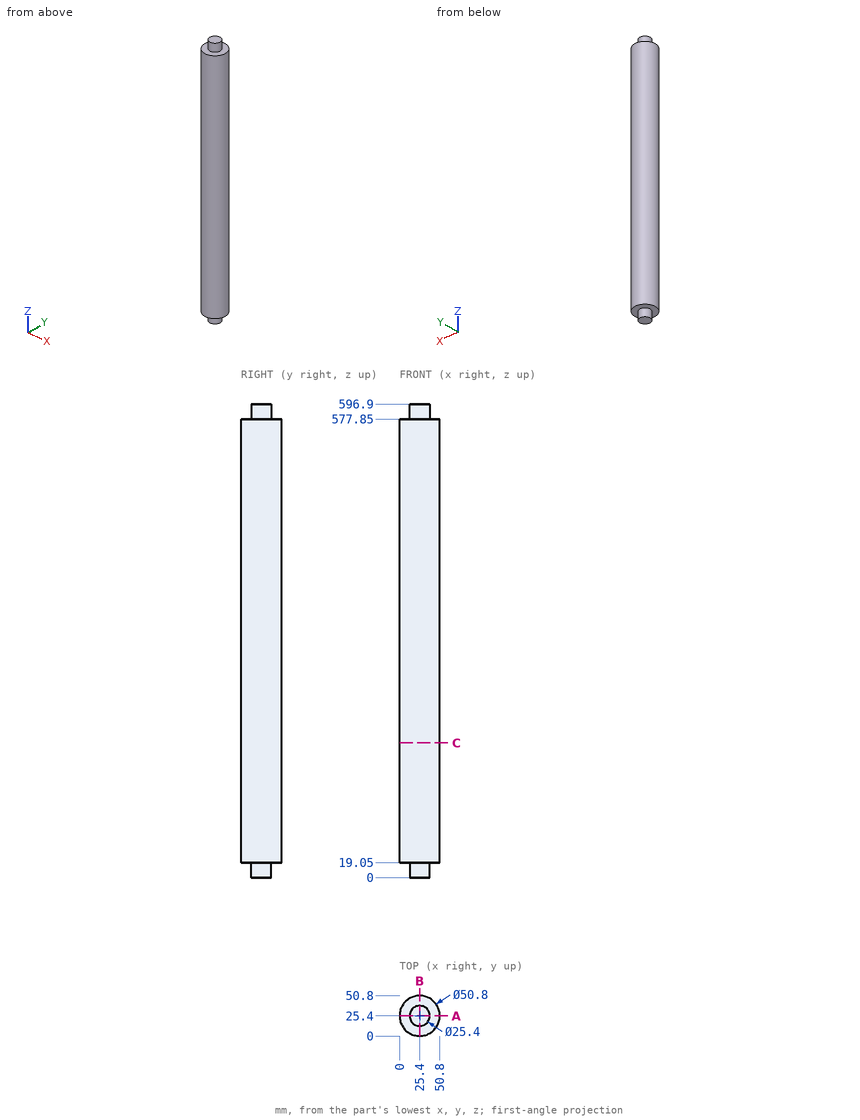
Study the drawing (mm; zero at the part's minimum x, y, z) and answer. Coordinates: 2 decimals unless noted, no trailing zeros. Write each loop counter-clockwise with the first axis right and the second up, starting at its lowest first coordinate (ties: lowest second). Pieces come first, ordered by that corner, then holes. Notation, with made-up numbers: M 87,18.25 L 137,18.25 A21 ccw 137,53.25 Z; hole C 60.5,84.25 d8. An arc over 180 degrees is marked long. Use a Markdown table: item, result. Add a question column.
1. Straight lines are drawn through the part: line 1 along X through (y, z) = (25, 227); line 2 along Z through (x, y) = (42, 22); line 3 along Y through (x, z) = (23.5, 475.5). For each, find the intervals that lie inside material, in ascending order. Write a range as [from, to].
2. Section C-C (z = 170) is taken. Give the vertices of the cut face in (x, y), plus the area to 3 significant figures.
3. Section A-A (y = 25.4) is taken. Give the vertices of the cut face in (x, z), plus the area to 3 significant figures.
4. Given P1, Ø12, axis at x = 7.5, y = 10, coming from the -Z side; P2, Ø6, axis at x = 35, z = 165.5, coming from the -Y side; P3, Ø12, axis at x = 27.5, z = 453, coming from the +Y side, each flat-ended and moving along its own axis, determine where each tip first touches the part or whether it passes through.
Data:
| question | item | result |
|---|---|---|
| 1 | line 1 | x = [0, 50.8] |
| 1 | line 2 | z = [19.05, 577.85] |
| 1 | line 3 | y = [0.07, 50.73] |
| 2 | outline | C 25.4,25.4 d50.8 |
| 2 | area | 2,030 mm2 |
| 3 | outline | M 0,19.05 L 12.7,19.05 L 12.7,0 L 38.1,0 L 38.1,19.05 L 50.8,19.05 L 50.8,577.85 L 38.1,577.85 L 38.1,596.9 L 12.7,596.9 L 12.7,577.85 L 0,577.85 Z |
| 3 | area | 29,400 mm2 |
| 4 | P1 | stops at z = 19.05 |
| 4 | P2 | stops at y = 0.87 |
| 4 | P3 | stops at y = 50.8 |
